Source: CAD feature listing. Evaluate the final solid. Frame: model axes, mm. Face numbers are marked on the shaded views. A direction names the side the tool comes from. Give positions to 0.01 mm unless a question says otherwise; leave off trailing zeros. Order: outer loops, then holes, each group sorted by start corner. A loop starts at its lowest first (then second) coordinate and runs counter-clockwise, first axis right, second up. Notation, with made-up numbers: M 28,46 L 60,46 A27 ccw 60,77 Z; hole C 20.5,89 d6. An arc over 180 degrees is marked long. Return JSON: item names as keys, results as strings.
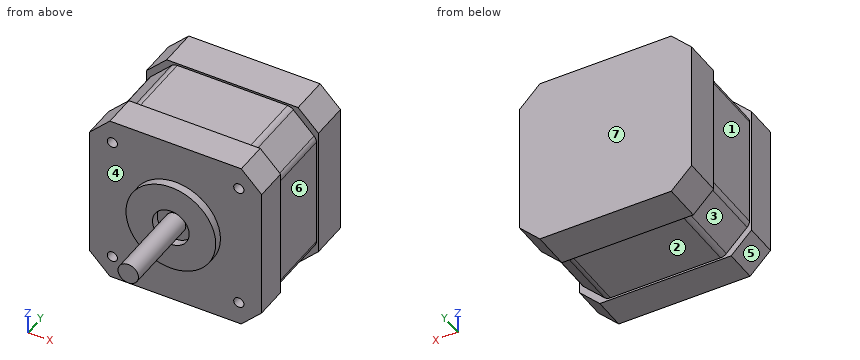
from build123d import *

# Parameters (mm, degrees)
F0_W      = 42.2
F0_H      = 42.2
F0_R      = 2.5
F1_DEPTH  = 33.3
F2_SIZE   = 5
F3_DEPTH  = 20
F4_R      = 11
F4_R_2    = 4.5
F5_DEPTH  = 2
F6_R      = 1.25
F7_DEPTH  = 5
F9_W      = 50.7564134896
F9_H      = 50.1955691725
F10_DEPTH = 16
F11_R     = 2


with BuildPart() as f1:
    # F0 (on Front) → F1 (new body)
    with BuildSketch(Plane.XZ):
        Rectangle(F0_W, F0_H)
        Circle(F0_R, mode=Mode.SUBTRACT)
        Circle(F0_R)
    extrude(amount=-F1_DEPTH)

    # F2
    f2_edges = [f1.edges().sort_by_distance(p)[0] for p in [
        (21.1, 16.65, 21.1),
        (-21.1, 16.65, 21.1),
        (21.1, 16.65, -21.1),
        (-21.1, 16.65, -21.1),
    ]]
    chamfer(f2_edges, length=F2_SIZE)

    # F0 (on Front) → F3 (join)
    with BuildSketch(Plane.XZ):
        Circle(F0_R)
    extrude(amount=F3_DEPTH)

    # F4 (on face) → F5 (join)
    with BuildSketch(Plane.XZ):
        Circle(F4_R)
        Circle(F4_R_2, mode=Mode.SUBTRACT)
    extrude(amount=F5_DEPTH)

    # F6 (on face) → F7 (cut)
    with BuildSketch(Plane.XZ):
        with Locations((-15.5, 15.5)):
            Circle(F6_R)
        with Locations((-15.5, -15.5)):
            Circle(F6_R)
        with Locations((15.5, -15.5)):
            Circle(F6_R)
        with Locations((15.5, 15.5)):
            Circle(F6_R)
    extrude(amount=-F7_DEPTH, mode=Mode.SUBTRACT)

    # F9 (on offset) → F10 (cut)
    with BuildSketch(Plane.XZ.offset(-8)):
        with Locations((0.5305930972, 0.0707069412)):
            Rectangle(F9_W, F9_H)
        Polygon((-14.3372583002, 20.6), (0, 20.6), (14.3372583002, 20.6), (20.6, 14.3372583002), (20.6, 0), (20.6, -14.3372583002), (14.3372583002, -20.6), (0, -20.6), (-14.3372583002, -20.6), (-20.6, -14.3372583002), (-20.6, 0), (-20.6, 14.3372583002), align=None, mode=Mode.SUBTRACT)
    extrude(amount=-F10_DEPTH, mode=Mode.SUBTRACT)

    # F11
    f11_edges = [f1.edges().sort_by_distance(p)[0] for p in [
        (20.6, 16, 14.337258),
        (14.337258, 16, 20.6),
        (-14.337258, 16, 20.6),
        (-20.6, 16, 14.337258),
        (-20.6, 16, -14.337258),
        (-14.337258, 16, -20.6),
        (20.6, 16, -14.337258),
        (14.337258, 16, -20.6),
    ]]
    fillet(f11_edges, radius=F11_R)


solid = f1.part
1. Section query D-D (z = 8.5). Return loops of the section in (x, y).
Evaluation:
{"outline": "M -21.1,0 L -6.98,0 L -6.98,-2 L 6.98,-2 L 6.98,0 L 21.1,0 L 21.1,8 L 20.6,8 L 20.6,24 L 21.1,24 L 21.1,33.3 L -21.1,33.3 L -21.1,24 L -20.6,24 L -20.6,8 L -21.1,8 Z"}
2. Section query A-A (y = 1.5). Return loops of the section in (x, z).
Evaluation:
{"outline": "M -21.1,-16.1 L -16.1,-21.1 L 16.1,-21.1 L 21.1,-16.1 L 21.1,16.1 L 16.1,21.1 L -16.1,21.1 L -21.1,16.1 Z; hole C -15.5,-15.5 d2.5; hole C -15.5,15.5 d2.5; hole C 15.5,-15.5 d2.5; hole C 15.5,15.5 d2.5"}
3. First-contact query: pin 1 (3 mm diameter, centred on x = 15.5, z = -15.5, fed in from -Y); pin 2 (6 mm diameter, centred on x = -7, y = 15.5, fed in from +Z); pin 3 (12 mm diameter, centred on x = -4.5, y = -11.5, fed in from +Z). Flat tips, straight axial feed; report the tip coordinate or a pass-through.
Evaluation:
{"pin 1": "stops at y = 0", "pin 2": "stops at z = 20.6", "pin 3": "stops at z = 2.5"}
4. Ray query, probe 1 along Z at (x, y) = (0, -1.35); probe 2 along Z at (x, y) = (15, 3); probe 3 along Y at (x, z) = (-17.5, -10.5). Return the intervals inside material, ascending.
Evaluation:
{"probe 1": "z = -11 to -4.5, -2.5 to 2.5, 4.5 to 11", "probe 2": "z = -21.1 to -16.65, -14.35 to 14.35, 16.65 to 21.1", "probe 3": "y = 0 to 33.3"}
5. Section query B-B (x = 0). Return loops of the section in (y, z).
Evaluation:
{"outline": "M -20,-2.5 L 0,-2.5 L 0,-4.5 L -2,-4.5 L -2,-11 L 0,-11 L 0,-21.1 L 8,-21.1 L 8,-20.6 L 24,-20.6 L 24,-21.1 L 33.3,-21.1 L 33.3,21.1 L 24,21.1 L 24,20.6 L 8,20.6 L 8,21.1 L 0,21.1 L 0,11 L -2,11 L -2,4.5 L 0,4.5 L 0,2.5 L -20,2.5 Z"}
6. Draft query along Y for the marked faces 5, 6 and 7. Return one class per face: pulls with the +Y half, pulls with the -Y half, needs draft (parallel to the pull), parting line crosses it, or undercut.
Evaluation:
{"face 5": "needs draft", "face 6": "undercut", "face 7": "pulls with the +Y half"}
7. Section query C-C (y = 30). Return loops of the section in (x, z).
Evaluation:
{"outline": "M -21.1,-16.1 L -16.1,-21.1 L 16.1,-21.1 L 21.1,-16.1 L 21.1,16.1 L 16.1,21.1 L -16.1,21.1 L -21.1,16.1 Z"}
8. Set-up query: the marked faces 1, 2, 3 and 4. Return all of +Z, -Z, +X, -X, +Y, -Y with unobstructed straight access to the full face (end or side cutting, diameter ignored); none if empty.
Evaluation:
{"face 1": "+Z, -Z, -X", "face 2": "-Z, +X, -X", "face 3": "-Z, -X", "face 4": "-Y"}
